from build123d import *

# Parameters (mm, degrees)
BOSS_EXTRUDE1_DEPTH             = 4.763
TAP_DRILL_FOR_M3X0_5_TAP1_D     = 2.5
TAP_DRILL_FOR_M3X0_5_TAP1_DEPTH = 5
TAP_DRILL_FOR_M3X0_5_TAP2_D     = 2.5
TAP_DRILL_FOR_M3X0_5_TAP2_DEPTH = 5


with BuildPart() as part:
    # Sketch2 → Boss-Extrude1 (new body)
    with BuildSketch(Plane(origin=(0, 0, 0), x_dir=(1, 0, 0), z_dir=(0, 1, 0))):
        Polygon((-66.5, -22.5), (118.5, -22.5), (118.5, 22.5), (113.5, 22.5), (59.963, 57.5), (16.213, 57.5), (-61.5, 22.5), (-66.5, 22.5), align=None)
        with BuildLine():
            Line((50.613, 49.325), (50.613, -14.325))
            ThreePointArc((50.613, -14.325), (47.438, -17.5), (44.263, -14.325))
            Line((44.263, -14.325), (44.263, 49.325))
            ThreePointArc((44.263, 49.325), (47.438, 52.5), (50.613, 49.325))
        make_face(mode=Mode.SUBTRACT)
        with BuildLine():
            Line((41.263, 49.325), (41.263, -14.325))
            ThreePointArc((41.263, -14.325), (38.088, -17.5), (34.913, -14.325))
            Line((34.913, -14.325), (34.913, 49.325))
            ThreePointArc((34.913, 49.325), (38.088, 52.5), (41.263, 49.325))
        make_face(mode=Mode.SUBTRACT)
        with BuildLine():
            Line((31.913, 49.325), (31.913, -14.325))
            ThreePointArc((31.913, -14.325), (28.738, -17.5), (25.563, -14.325))
            Line((25.563, -14.325), (25.563, 49.325))
            ThreePointArc((25.563, 49.325), (28.738, 52.5), (31.913, 49.325))
        make_face(mode=Mode.SUBTRACT)
        with BuildLine():
            Line((59.963, 49.325), (59.963, -14.325))
            ThreePointArc((59.963, -14.325), (56.788, -17.5), (53.613, -14.325))
            Line((53.613, -14.325), (53.613, 49.325))
            ThreePointArc((53.613, 49.325), (56.788, 52.5), (59.963, 49.325))
        make_face(mode=Mode.SUBTRACT)
        with BuildLine():
            Line((22.563, 49.325), (22.563, -14.325))
            ThreePointArc((22.563, -14.325), (19.388, -17.5), (16.213, -14.325))
            Line((16.213, -14.325), (16.213, 49.325))
            ThreePointArc((16.213, 49.325), (19.388, 52.5), (22.563, 49.325))
        make_face(mode=Mode.SUBTRACT)
        with BuildLine():
            Line((-59.6842053, 17.076061462), (-29.0027053, 12.617481945))
            ThreePointArc((-29.0027053, 12.617481945), (-28.030463852, 12.085169259), (-27.6435, 11.04648297))
            Line((-27.6435, 11.04648297), (-27.6435, 8.800559076))
            ThreePointArc((-27.6435, 8.800559076), (-28.033123359, 7.758806801), (-29.010741325, 7.228413292))
            Line((-29.010741325, 7.228413292), (-59.692241325, 2.929914643))
            ThreePointArc((-59.692241325, 2.929914643), (-60.954252275, 3.304183785), (-61.5, 4.502060427))
            Line((-61.5, 4.502060427), (-61.5, 15.505062487))
            ThreePointArc((-61.5, 15.505062487), (-60.951186289, 16.705598635), (-59.6842053, 17.076061462))
        make_face(mode=Mode.SUBTRACT)
        with BuildLine():
            Line((-59.680570174, -2.76869727), (-28.999070174, -7.299806511))
            ThreePointArc((-28.999070174, -7.299806511), (-28.029262747, -7.832976538), (-27.6435, -8.87027294))
            Line((-27.6435, -8.87027294), (-27.6435, -11.12972706))
            ThreePointArc((-27.6435, -11.12972706), (-28.029262747, -12.167023462), (-28.999070174, -12.700193489))
            Line((-28.999070174, -12.700193489), (-59.680570174, -17.23130273))
            ThreePointArc((-59.680570174, -17.23130273), (-60.949796402, -16.862573553), (-61.5, -15.6608363))
            Line((-61.5, -15.6608363), (-61.5, -4.3391637))
            ThreePointArc((-61.5, -4.3391637), (-60.949796402, -3.137426447), (-59.680570174, -2.76869727))
        make_face(mode=Mode.SUBTRACT)
        with BuildLine():
            Line((-22.6435, -8.87027294), (-22.6435, -11.12972706))
            ThreePointArc((-22.6435, -11.12972706), (-22.257737253, -12.167023462), (-21.287929826, -12.700193489))
            Line((-21.287929826, -12.700193489), (9.393570174, -17.23130273))
            ThreePointArc((9.393570174, -17.23130273), (10.662796402, -16.862573553), (11.213, -15.6608363))
            Line((11.213, -15.6608363), (11.213, -4.3391637))
            ThreePointArc((11.213, -4.3391637), (10.662796402, -3.137426447), (9.393570174, -2.76869727))
            Line((9.393570174, -2.76869727), (-21.287929826, -7.299806511))
            ThreePointArc((-21.287929826, -7.299806511), (-22.257737253, -7.832976538), (-22.6435, -8.87027294))
        make_face(mode=Mode.SUBTRACT)
        with BuildLine():
            Line((-22.6435, 8.79344646), (-22.6435, 11.04648297))
            ThreePointArc((-22.6435, 11.04648297), (-22.256536148, 12.085169259), (-21.2842947, 12.617481945))
            Line((-21.2842947, 12.617481945), (9.3972053, 17.076061462))
            ThreePointArc((9.3972053, 17.076061462), (10.664186289, 16.705598635), (11.213, 15.505062487))
            Line((11.213, 15.505062487), (11.213, 4.334866943))
            ThreePointArc((11.213, 4.334866943), (10.664186289, 3.134330795), (9.3972053, 2.763867968))
            Line((9.3972053, 2.763867968), (-21.2842947, 7.222447484))
            ThreePointArc((-21.2842947, 7.222447484), (-22.256536148, 7.754760171), (-22.6435, 8.79344646))
        make_face(mode=Mode.SUBTRACT)
        with BuildLine():
            Line((64.963, 15.499376461), (64.963, 4.486336964))
            ThreePointArc((64.963, 4.486336964), (65.559394235, 3.246229867), (66.900468488, 2.93789313))
            Line((66.900468488, 2.93789313), (85.493968488, 7.140266464))
            ThreePointArc((85.493968488, 7.140266464), (86.384107097, 7.697604533), (86.7315, 8.688710298))
            Line((86.7315, 8.688710298), (86.7315, 11.160279322))
            ThreePointArc((86.7315, 11.160279322), (86.387560859, 12.147048109), (85.504775415, 12.706240948))
            Line((85.504775415, 12.706240948), (66.911275415, 17.045338087))
            ThreePointArc((66.911275415, 17.045338087), (65.563731213, 16.74293732), (64.963, 15.499376461))
        make_face(mode=Mode.SUBTRACT)
        with BuildLine():
            Line((91.7315, 11.160279322), (91.7315, 8.688710298))
            ThreePointArc((91.7315, 8.688710298), (92.078892903, 7.697604533), (92.969031512, 7.140266464))
            Line((92.969031512, 7.140266464), (113.5, 2.5))
            Line((113.5, 2.5), (113.5, 15.499376461))
            ThreePointArc((113.5, 15.499376461), (112.899268787, 16.74293732), (111.551724585, 17.045338087))
            Line((111.551724585, 17.045338087), (92.958224585, 12.706240948))
            ThreePointArc((92.958224585, 12.706240948), (92.075439141, 12.147048109), (91.7315, 11.160279322))
        make_face(mode=Mode.SUBTRACT)
        with BuildLine():
            Line((86.7315, -8.764205555), (86.7315, -11.235794445))
            ThreePointArc((86.7315, -11.235794445), (86.385837257, -12.22473149), (85.499378453, -12.783005615))
            Line((85.499378453, -12.783005615), (66.905878453, -17.053740852))
            ThreePointArc((66.905878453, -17.053740852), (65.561562955, -16.748366938), (64.963, -15.506529682))
            Line((64.963, -15.506529682), (64.963, -4.493470318))
            ThreePointArc((64.963, -4.493470318), (65.561562955, -3.251633062), (66.905878453, -2.946259148))
            Line((66.905878453, -2.946259148), (85.499378453, -7.216994385))
            ThreePointArc((85.499378453, -7.216994385), (86.385837257, -7.77526851), (86.7315, -8.764205555))
        make_face(mode=Mode.SUBTRACT)
        with BuildLine():
            Line((91.7315, -8.764205555), (91.7315, -11.235794445))
            ThreePointArc((91.7315, -11.235794445), (92.077162743, -12.22473149), (92.963621547, -12.783005615))
            Line((92.963621547, -12.783005615), (111.557121547, -17.053740852))
            ThreePointArc((111.557121547, -17.053740852), (112.901437045, -16.748366938), (113.5, -15.506529682))
            Line((113.5, -15.506529682), (113.5, -4.493470318))
            ThreePointArc((113.5, -4.493470318), (112.901437045, -3.251633062), (111.557121547, -2.946259148))
            Line((111.557121547, -2.946259148), (92.963621547, -7.216994385))
            ThreePointArc((92.963621547, -7.216994385), (92.077162743, -7.77526851), (91.7315, -8.764205555))
        make_face(mode=Mode.SUBTRACT)
    extrude(amount=BOSS_EXTRUDE1_DEPTH)

    # Tap Drill for M3x0.5 Tap1
    with Locations(Plane(origin=(118.5, 0, 0), x_dir=(0, 0, -1), z_dir=(1, 0, 0))):
        with Locations((-11.25, 2.3815), (11.25, 2.3815)):
            Hole(TAP_DRILL_FOR_M3X0_5_TAP1_D / 2, depth=TAP_DRILL_FOR_M3X0_5_TAP1_DEPTH)

    # Tap Drill for M3x0.5 Tap2
    with Locations(Plane.ZY.offset(66.5)):
        with Locations((11.25, 2.3815), (-11.25, 2.3815)):
            Hole(TAP_DRILL_FOR_M3X0_5_TAP2_D / 2, depth=TAP_DRILL_FOR_M3X0_5_TAP2_DEPTH)


solid = part.part
Can you work these out from the model? Positions are in its coordinate system, mm. A direction names the side the tool comes from. Give positions to 0.01 mm unless a question says otherwise; leave off trailing zeros. Order: outer loops, then holes, each group sorted by start corner. A loop starts at its lowest first (then second) coordinate and runs counter-clockwise, first axis right, second up. Notation, with made-up numbers: (2, 11) - (24, 11) arc R14 ccw to (24, 24) - close; hole circle Ø3 at (29, 72.5). An arc over 180 degrees is marked (long way). Write each question's results on one line, items separated by ' | '.
1) Suppose I cut it at A-A, the plane z = -19. Write out the boundary of the cut face in (x, y).
Final values:
outline: (-66.5, 0) - (16.21, 0) - (16.21, 4.76) - (-66.5, 4.76) - close; (22.56, 0) - (25.56, 0) - (25.56, 4.76) - (22.56, 4.76) - close; (31.91, 0) - (34.91, 0) - (34.91, 4.76) - (31.91, 4.76) - close; (41.26, 0) - (44.26, 0) - (44.26, 4.76) - (41.26, 4.76) - close; (50.61, 0) - (53.61, 0) - (53.61, 4.76) - (50.61, 4.76) - close; (59.96, 0) - (118.5, 0) - (118.5, 4.76) - (59.96, 4.76) - close
2) Please list where these lines run through material, in increasing order: line 1 along X through (y, z) = (3.8, -20.5); line 2 along Y through (x, z) = (-62, -11); line 3 along X through (y, z) = (0.8, -38). Write a range as [from, to].
Final values:
line 1: x = [-66.5, 16.21], [22.56, 25.56], [31.91, 34.91], [41.26, 44.26], [50.61, 53.61], [59.96, 118.5] | line 2: y = [0, 1.16], [3.61, 4.76] | line 3: x = [-27.08, 16.21], [22.56, 25.56], [31.91, 34.91], [41.26, 44.26], [50.61, 53.61], [59.96, 89.79]
3) Suppose I cut it at D-D, the plane x = 104. Write out the boundary of the cut face in (y, z), then the cut area to 3 significant figures.
Final values:
outline: (0, -28.71) - (4.76, -28.71) - (4.76, -15.28) - (0, -15.28) - close; (0, -4.65) - (4.76, -4.65) - (4.76, 4.68) - (0, 4.68) - close; (0, 15.32) - (4.76, 15.32) - (4.76, 22.5) - (0, 22.5) - close | area: 143 mm^2
4) On a 3-axis mill with a long thin cutter (end or side, diameter ignored), from which of +Z, -Z, +X, -X, +Y, -Y can I reach the whole of each face in a straight line? I mean faces 5 (the face through (-66.5, 2, 0)), 6 (the face through (44.263, 2, -17)). Say none if no direction works.
Final values:
face 5: +Z, -Z, -X, +Y, -Y | face 6: +Y, -Y
5) Suppose I cut it at C-C, the plane z = -31.5. Write out the boundary of the cut face in (x, y).
Final values:
outline: (-41.52, 0) - (16.21, 0) - (16.21, 4.76) - (-41.52, 4.76) - close; (22.56, 0) - (25.56, 0) - (25.56, 4.76) - (22.56, 4.76) - close; (31.91, 0) - (34.91, 0) - (34.91, 4.76) - (31.91, 4.76) - close; (41.26, 0) - (44.26, 0) - (44.26, 4.76) - (41.26, 4.76) - close; (50.61, 0) - (53.61, 0) - (53.61, 4.76) - (50.61, 4.76) - close; (59.96, 0) - (99.73, 0) - (99.73, 4.76) - (59.96, 4.76) - close
6) Suppose I cut it at B-B, the plane x = -5. Write out the boundary of the cut face in (y, z).
Final values:
outline: (0, -47.95) - (4.76, -47.95) - (4.76, -14.98) - (0, -14.98) - close; (0, -4.86) - (4.76, -4.86) - (4.76, 4.89) - (0, 4.89) - close; (0, 15.11) - (4.76, 15.11) - (4.76, 22.5) - (0, 22.5) - close
7) If we mould it in two halves opening along X, with no side actions, what happens to faces 1 (the face through (116, 2, -22.5)), 2 (the face through (-22.1, 2.348, -40.245)), 3 (the face through (76.07, 2.35, -5.01)), 4 (the face through (25.563, 2, -17))? For each: pulls with the +X half, pulls with the -X half, needs draft (parallel to the pull), parting line crosses it, or undercut.
Final values:
face 1: needs draft | face 2: pulls with the -X half | face 3: undercut | face 4: undercut
8) I'm going to push flat-ended pins straight in: pin 1 Ø8 at (x, z) = (-47, 9) entering from +Y; pin 2 Ø2.5 at (y, z) = (1.5, -10.5) entering from +X; pin 3 Ø1.5 at (y, z) = (2.38, 11.25) entering from -X; pin 4 Ø1.4 at (y, z) = (2.5, -29) entering from +X. Where does each tip first touch, or does it pass through?
Final values:
pin 1: passes through | pin 2: stops at x = 118.5 | pin 3: stops at x = -27.9 | pin 4: stops at x = 104.63
